Source: CAD feature listing. Evaluate the final solid. Frame: model axes, mm. Face numbers are marked on the shaded views. A direction names the side the tool comes from. Give positions to 0.01 mm unless a question says otherwise; leave off trailing zeros. Loops run counter-clockwise (first coordinate to the right, second up) from the corner with the lowest first, then second, coordinate; pieces in that order, holes last.
Autodesk Inventor part; units mm, degrees
ref_plane "YZ Plane" through (0, 0, 0) normal (1, 0, 0) x (0, 1, 0)
ref_plane "XZ Plane" through (0, 0, 0) normal (0, 1, 0) x (-1, 0, 0)
ref_plane "XY Plane" through (0, 0, 0) normal (0, 0, 1) x (1, 0, 0)
sketch "Sketch1" plane through (0, 0, 0) normal (0, 0, 1) x (1, 0, 0)
  circle A0 centre (0, 0) radius 2.413
  dimension "d0" = 4.826
extrude "Extrusion1" add sketch "Sketch1" along normal blind 22.225
sketch "Sketch2" plane through (0, 0, 0) normal (0, 1, 0) x (-1, 0, 0)
  line L0 (0, 0) -> (0, -2.5654)
  line L1 (0, 0) -> (4.3239, 0)
  line L2 (0, -2.5654) -> (2.032, -2.5654)
  line L3 (4.3239, 0) -> (4.3239, 3.8864) construction
  arc A0 (4.5568, -0.3781) -> (4.3239, 0) centre (4.3239, -0.2608) ccw
  arc A1 (2.032, -2.5654) -> (4.5568, -0.3781) centre (0.6382, 1.5944) ccw
  line L4 (4.5847, 0.6553) -> (4.5847, -0.2608) construction
  dimension "d3" = 2.5654
  dimension "d6" = 2.032
  dimension "d12" = 4.5847
revolve "Revolution1" add sketch "Sketch2" angle 360 about axis through (0, 0, 0) along (0, 0, -1)
sketch "Sketch3" plane through (0, 0, -2.5654) normal (0, 0, -1) x (-1, 0, 0)
  circle A0 centre (0, 0) radius 2.032
  line L0 (-0.9165, 1.5875) -> (0.9165, 1.5875)
  line L1 (0.9165, 1.5875) -> (1.8331, 0)
  line L2 (1.8331, 0) -> (0.9165, -1.5875)
  line L3 (0.9165, -1.5875) -> (-0.9165, -1.5875)
  line L4 (-0.9165, -1.5875) -> (-1.8331, 0)
  line L5 (-1.8331, 0) -> (-0.9165, 1.5875)
  dimension "d8" = 3.175
extrude "Extrusion2" cut sketch "Sketch3" against normal blind 1.5875 contours L0 L1 L2 L3 L4 L5
chamfer "Chamfer1" distance 0.508 angle 45 1 edges at (-2.413, 0, 22.225)
thread "Thread1"
properties part number "10-32 x625 button head" material "Steel"
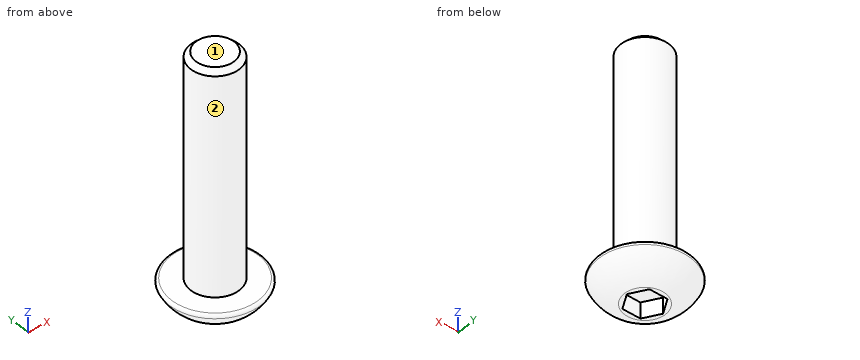
1) Reachability of the marked faces 1 and 2 from +Z, -Z, +X, -X, +Y, -Y: full face, straight path, thin tool, end or side. Return the list, or none.
Checks:
face 1: +Z, +X, -X, +Y, -Y
face 2: +Z
2) Contact query for flat-ended pins moving along their axis: P1, Ø2.5, axis at x = 0, y = 0, coming from the -Z side; P2, Ø1.5, axis at y = 1, z = 7, coming from the -X side; P3, Ø3, axis at x = 1.5, z = 12, coming from the +Y side. Output: stop coordinate, or through.
Checks:
P1: stops at z = -0.98
P2: stops at x = -2.4
P3: stops at y = 2.41
3) Cut plane A-A (z = 19). Return loops of the section in (x, y).
Checks:
outline: circle Ø4.83 at (0, 0)
4) Ray query, probe 1 along Y at (x, z) = (0, 3.5); probe 2 along X at (y, z) = (-1.75, 4.25); probe 3 along Z at (x, y) = (-0.75, -3). Return the intervals inside material, ascending.
Checks:
probe 1: y = -2.41 to 2.41
probe 2: x = -1.66 to 1.66
probe 3: z = -2.04 to 0
